For this review, use the dimensioned drawing (mm, ordinates from the lowest corner) and the shaded views. A direction names the side the tool comes from. Give positions to 0.01 mm unless a question says otherwise; leave off trailing zeros. Write each loop counter-clockwise with the first axis right and the second up, starting at its lowest first coordinate (ties: lowest second). Pieces come first, ordered by that corner, then holes. Notation, with made-up numbers: M -5.75,58 L 49.25,58 A22 ccw 49.25,72 Z; hole C -30,-14 d11. An arc over 180 degrees is marked long. Write each question's results on one line, items separated by ' | '. Start each with the question number.
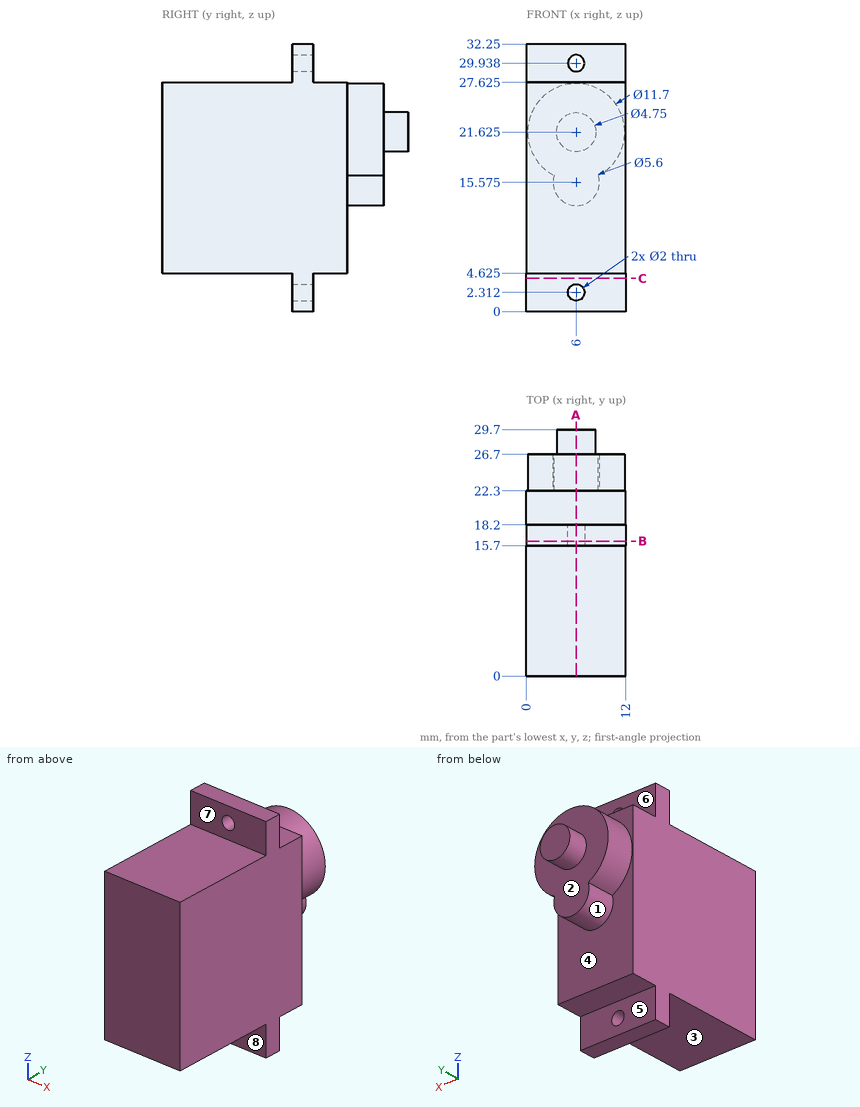
(1) Add section B-B (y = 16.25). State the section outline as (x, z) points.
(2) Add section A-A (x = 6). Give the number of separate pieces and of enclosed holes in the cut face, then the cut area to 3 significant figures.
(3) Machinability: for the marked faces 4, 5, 6, 7 and 8, which of the approach directions +Z, -Z, +X, -X, +Y, -Y give a long, thin tool a straight path to every point of the face, cutting with its end or side? Answer none if there is none.
(4) Clearance check with flat-ended pins moving along their axes: P1, Ø3.5, axis at x = 6, z = 2.5, coming from the +Y side; P2, Ø6, axis at x = 5, y = 12, coming from the +Z side (1 decimal); P3, Ø4, axis at x = 4.5, z = 27, coming from the +Y side. State where each tip first meets the part, or that it passes through.
(5) Add section C-C (z = 4). State the section outline as (x, y) points, then the cut area to 3 significant figures.
(6) Wall thickness on L1, parallel to Z at x = 6, y = 17.6; L2, parallel to Y at x = 9.75, z = 7; L3, parallel to Z at x = 1.5, y = 4 (1 decimal): over which ranges is each line inside the solid? List them lowest first.
(7) Draft analysis for pull direction Z (two halves, no side actions). For the marked faces 1, 2 and 3, state which applies: pulls with the +Z half, pulls with the -Z half, needs draft (parallel to the pull), parting line crosses it, or undercut.
Calculated:
1) outline: M 0,0 L 12,0 L 12,32.25 L 0,32.25 Z; hole C 6,2.31 d2; hole C 6,29.94 d2
2) separate pieces: 3 | enclosed holes: 0 | area: 605 mm²
3) face 4: +Y | face 5: -Z, +X, -X, +Y | face 6: +Z, +X, -X, +Y | face 7: +Z, +X, -X, -Y | face 8: -Z, +X, -X, -Y
4) P1: stops at y = 18.2 | P2: stops at z = 27.6 | P3: stops at y = 26.7
5) outline: M 0,15.7 L 12,15.7 L 12,18.2 L 0,18.2 Z | area: 30.0 mm²
6) L1: z = 0 to 1.31, 3.31 to 28.94, 30.94 to 32.25 | L2: y = 0 to 22.3 | L3: z = 4.6 to 27.6
7) face 1: undercut | face 2: needs draft | face 3: pulls with the -Z half
